CAD build for the part. Positions are in the model's coordinates, mm. Round coordinates to 2 decimals unless told otherwise and drop trailing zeros. Order: outer loops, then holes, each group sorted by start corner. A loop starts at its lowest first (then second) coordinate and runs counter-clockwise, first axis right, second up. Notation, with made-up numbers: (-22, 34.5) -> (-7, 34.5) arc R13 ccw to (-7, 53.5) -> close; hole circle Ø10 at (73, -31). An arc over 180 degrees is marked (long way). Return JSON: item names as keys, results as strings. Group by question number.
Q1. Cut at A-A (y = 0). Write the cut outline in (x, z), then the cut area to 3 significant figures.
Q2. Mould opens along Y. For faces 1 (the cylindrical face through (-1.38, -6.2, 0.79)), 2 (the flat face through (5, -5, 1.588)), 3 (the cylindrical face through (-2.75, -12.4, 0.79)) say: +Y half, -Y half, draft (parallel to the pull), parting line (faces both ways), or undercut.
Q3. Cut at C-C (z = 0.9). Write the cut outline in (x, y), then the cut area to 3 significant figures.
Q4. Probe line 1 along Y through (x, z) = (0, 0.95); line 2 along Y through (x, z) = (4.75, 1.15); line 3 along X through (y, z) = (3.25, 0.1). List the from-to ranges inside material, lowest first.
from build123d import *

# Parameters (mm, degrees)
F0_R     = 12.7
F0_R_2   = 6.35
F1_DEPTH = 1.5875
F2_R     = 0.396875


with BuildPart() as f1:
    # F0 (on Top) → F1 (new body)
    with BuildSketch(Plane.XY):
        Circle(F0_R)
        Circle(F0_R_2, mode=Mode.SUBTRACT)
    extrude(amount=F1_DEPTH)

    # F2
    f2_edges = [f1.edges().sort_by_distance(p)[0] for p in [
        (-12.7, 0, 0),
        (-6.35, 0, 0),
        (-12.7, 0, 1.5875),
        (12.7, 0, 0.79375),
        (-6.35, 0, 1.5875),
        (6.35, 0, 0.79375),
    ]]
    fillet(f2_edges, radius=F2_R)


solid = f1.part
Solution:
{
 "1": {"outline": "(-12.7, 0.4) arc R0.4 ccw to (-12.3, 0) -> (-6.75, 0) arc R0.4 ccw to (-6.35, 0.4) -> (-6.35, 1.19) arc R0.4 ccw to (-6.75, 1.59) -> (-12.3, 1.59) arc R0.4 ccw to (-12.7, 1.19) -> close; (6.35, 0.4) arc R0.4 ccw to (6.75, 0) -> (12.3, 0) arc R0.4 ccw to (12.7, 0.4) -> (12.7, 1.19) arc R0.4 ccw to (12.3, 1.59) -> (6.75, 1.59) arc R0.4 ccw to (6.35, 1.19) -> close", "area": "19.9 mm²"},
 "2": {"face 1": "undercut", "face 2": "draft", "face 3": "parting line"},
 "3": {"outline": "circle Ø25.4 at (0, 0); hole circle Ø12.7 at (0, 0)", "area": "380 mm²"},
 "4": {"line 1": "y = -12.7 to -6.35, 6.35 to 12.7", "line 2": "y = -11.78 to -4.21, 4.21 to 11.78", "line 3": "x = -12.14 to -5.61, 5.61 to 12.14"}
}
